For this review, take the finished solid that the model builds, in its own axes (mm). A direction names the side the tool comes from. Coordinates: 2 decimals unless noted, no trailing zeros. Write each loop counter-clockwise with the first axis right and the second up, starting at its lowest first coordinate (ties: lowest second). Pieces come first, ordered by that corner, then holes. Notation, with made-up numbers: M 9.5,68 L 28.5,68 A17 ccw 28.5,94 Z; hole C -22.75,74.25 d9. An arc over 180 degrees is marked long. Return JSON: item names as keys, results as strings.
Autodesk Inventor part; units mm, degrees
ref_plane "YZ Plane" through (0, 0, 0) normal (1, 0, 0) x (0, 1, 0)
ref_plane "XZ Plane" through (0, 0, 0) normal (0, 1, 0) x (-1, 0, 0)
ref_plane "XY Plane" through (0, 0, 0) normal (0, 0, 1) x (1, 0, 0)
sketch "Sketch1" plane through (0, 0, 0) normal (0, 0, 1) x (1, 0, 0)
  circle A0 centre (0, 0) radius 28.575
  dimension "d0" = 57.15
extrude "Extrusion1" add sketch "Sketch1" along normal blind 4.572
sketch "Sketch2" plane through (0, 0, 4.572) normal (0, 0, 1) x (1, 0, 0)
  circle A0 centre (0, 0) radius 28.575
  circle A1 centre (0, 0) radius 12.1666
  dimension "d3" = 24.3332
extrude "Extrusion2" add sketch "Sketch2" along normal blind 20.828 contours A1
sketch "Sketch3" plane through (0, 0, 25.4) normal (0, 0, 1) x (1, 0, 0)
  circle A0 centre (0, 0) radius 12.1666
  circle A1 centre (0, 0) radius 6.35
  line L0 (-1.5875, 7.7359) -> (1.5875, 7.7359)
  line L1 (1.5875, 7.7359) -> (1.5875, 4.5609)
  line L2 (1.5875, 4.5609) -> (-1.5875, 4.5609)
  line L3 (-1.5875, 4.5609) -> (-1.5875, 7.7359)
  point P0 (0, 7.7359)
  point P1 (-1.5875, 6.1484)
  dimension "d6" = 12.7
  dimension "d7" = 3.175
  dimension "d8" = 3.175
extrude "Extrusion3" cut sketch "Sketch3" against normal through all contours A1 L3 L2 L1 | L1 L2 L3 A1 | A1 L3 L0 L1
sketch "Sketch4" plane through (0, 0, 0) normal (0, 0, -1) x (-1, 0, 0)
  arc A0 (-1.5875, 6.1484) -> (1.5875, 6.1484) centre (0, 0) ccw construction
  circle A1 centre (0, 0) radius 28.575 construction
  circle A2 centre (0, 0) radius 23.8125 construction
  point P0 (0, 23.8125)
  dimension "d11" = 47.625
hole "Hole1" at (0, 23.8125, 0) direction (0, 0, 1) diameter 5.1816 end through all
pattern_circular "Circular Pattern1" count 6 over 360 about axis through (0, 0, 0) along (0, 0, 1) of "Hole1"
properties part number "Hub 500 key" material "Aluminum 6061"
1. For faces 1 (the face through (-2, -12, 15)), 2 (the face through (5, -5, 25.4)), 3 (the face through (0, 7.736, 13)), list the 3-axis set-ups (+Z, -Z, +X, -X, +Y, -Y) from which the entire face can be reached by the end or side of a thin tool; tool diameter is ignored.
Checks:
{"face 1": "+Z", "face 2": "+Z, +X, -X, +Y, -Y", "face 3": "+Z, -Z"}
2. Wall thickness on L1, parallel to Y at x = 0, z = 6.25; L2, parallel to Y at x = 21.5, z = 2; L3, parallel to Z at x = -20, y = -5: over which ranges is each line inside the solid? List them lowest first. Write a range as from..to.
Checks:
{"L1": "-12.17..-6.35, 7.74..12.17", "L2": "-18.82..-14.34, -9.47..9.47, 14.34..18.82", "L3": "0..4.57"}
3. Draft analysis for pull direction X (two halves, no side actions). For faces 4 (the face through (1.588, 7, 13)), 5 (the face through (-28.547, -1.256, 2.254)), 6 (the face through (-7, 0, 0)), state which applies: +X half, -X half, draft (parallel to the pull), parting line (faces both ways), or undercut.
Checks:
{"face 4": "undercut", "face 5": "parting line", "face 6": "draft"}
4. We need section B-B (x = 0). State the section outline as (y, z) points (3 decimals), plus the area to 3 significant figures.
Checks:
{"outline": "M -28.575,0 L -26.403,0 L -26.403,4.572 L -28.575,4.572 Z; M -21.222,0 L -6.35,0 L -6.35,25.4 L -12.167,25.4 L -12.167,4.572 L -21.222,4.572 Z; M 7.736,0 L 21.222,0 L 21.222,4.572 L 12.167,4.572 L 12.167,25.4 L 7.736,25.4 Z; M 26.403,0 L 28.575,0 L 28.575,4.572 L 26.403,4.572 Z", "area": "363 mm2"}
5. We need section C-C (z = 14.75). State the section outline as (x, y) points, plus the area to 3 significant figures.
Checks:
{"outline": "C 0,0 d24.33; hole M -1.59,6.15 A6.35 ccw long 1.59,6.15 L 1.59,7.74 L -1.59,7.74 Z", "area": "334 mm2"}
6. We need section D-D (y = 10.5). State the section outline as (x, z) points, plus the area to 3 significant figures.
Checks:
{"outline": "M -26.58,0 L -22.8,0 L -22.8,4.57 L -26.58,4.57 Z; M -18.45,0 L 18.45,0 L 18.45,4.57 L 6.15,4.57 L 6.15,25.4 L -6.15,25.4 L -6.15,4.57 L -18.45,4.57 Z; M 22.8,0 L 26.58,0 L 26.58,4.57 L 22.8,4.57 Z", "area": "459 mm2"}
7. We need section A-A (y = 0). State the section outline as (x, z) points (3 decimals).
Checks:
{"outline": "M -28.575,0 L -6.35,0 L -6.35,25.4 L -12.167,25.4 L -12.167,4.572 L -28.575,4.572 Z; M 6.35,0 L 28.575,0 L 28.575,4.572 L 12.167,4.572 L 12.167,25.4 L 6.35,25.4 Z"}
8. Clearance check with flat-ended pins moving along their axes: pin 1 Ø10 at (x, y) = (-17.5, 14) entering from +Z; pin 2 Ø1.7 at (y, z) = (7, 10) entering from -X; pin 3 Ø3.5 at (x, z) = (-0.5, 8) entering from -Y. State where each tip first meets the part, or that it passes through.
Checks:
{"pin 1": "z = 4.57", "pin 2": "x = -10.5", "pin 3": "y = -12.17"}
